Input: part model. Units: mm. Frame: model coordinates. Face numbers are marked on the shaded views. A direction names the side the tool comes from. Round coordinates to 2 decimals unless told otherwise and drop trailing zeros. Write each loop counter-clockwise with the first axis right and the second up, starting at its lowest first coordinate (ties: lowest second). Pieces come first, ordered by that corner, then holes. Notation, with made-up numbers: (41, 43) -> (48, 43) arc R31 cw to (48, 67) -> close; hole circle Ø7 at (53.5, -21.75). An arc over 180 degrees is marked (long way). Use CSV: the item, a comma, the result in double quotes.
```python
from build123d import *

# Parameters (mm, degrees)
SALIENTE_EXTRUIR1_DEPTH = 25.4
SALIENTE_EXTRUIR2_DEPTH = 12.7
CROQUIS4_R              = 3.96875
CORTAR_EXTRUIR2_DEPTH   = 143.085809608
REDONDEO1_SIZE          = 6.35


with BuildPart() as part:
    # Croquis1 → Saliente-Extruir1 (new, symmetric)
    with BuildSketch(Plane.XY):
        Polygon((21.5228, 45.6639), (31.367398371, 8.254586189), (0, 0), (-20, -40), (-123, -40), (-125, -38.012905156), (-125, -12.012905156), (-123.000083272, -10), (-65.000083272, -10), (-65.000083272, 15), (-107.993526537, 15), (-110, 16.993526537), (-110, 37.993526537), (-108.006473463, 40), (0, 40), align=None)
    extrude(amount=SALIENTE_EXTRUIR1_DEPTH, both=True)

    # Croquis2 → Saliente-Extruir2 (add, symmetric)
    with BuildSketch(Plane.XY):
        Polygon((29.677177015, 14.677399874), (92.537004524, 31.219530495), (86.072848866, 55.783216937), (23.213021357, 39.241086316), align=None)
    extrude(amount=SALIENTE_EXTRUIR2_DEPTH, both=True)

    # Croquis4 → Cortar-Extruir2 (cut, through all)
    with BuildSketch(Plane.XY.offset(12.7)):
        with Locations((72.381126981, 39.047723164)):
            Circle(CROQUIS4_R)
        with Locations((43.3688989, 31.412893647)):
            Circle(CROQUIS4_R)
    extrude(amount=-CORTAR_EXTRUIR2_DEPTH, mode=Mode.SUBTRACT)

    # Redondeo1
    redondeo1_edges = [part.edges().sort_by_distance(p)[0] for p in [
        (61.107090769, 22.948465184, -12.7),
        (54.642935111, 47.512151626, -12.7),
        (61.107090769, 22.948465184, 12.7),
        (54.642935111, 47.512151626, 12.7),
    ]]
    chamfer(redondeo1_edges, length=REDONDEO1_SIZE)


solid = part.part
```
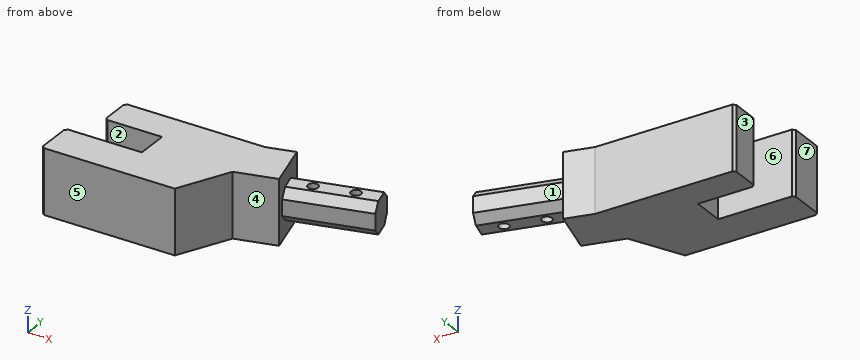
Item 1: Section query C-C on z = 16.5. Return the cut outline in (x, y), plus the area to 3 significant figures.
Worked answers:
outline,"(-125, -38.01) -> (-123, -40) -> (-20, -40) -> (0, 0) -> (31.37, 8.25) -> (21.52, 45.66) -> (0, 40) -> (-108.01, 40) -> (-110, 37.99) -> (-110, 16.99) -> (-107.99, 15) -> (-65, 15) -> (-65, -10) -> (-123, -10) -> (-125, -12.01) -> close"
area,"8,770 mm²"
Item 2: Section query D-D on x = 43. Return the cut outline in (y, z).
Worked answers:
outline,"(18.18, -6.35) -> (24.75, -12.7) -> (27.46, -12.7) -> (27.46, 12.7) -> (24.75, 12.7) -> (18.18, 6.35) -> close; (35.36, -12.7) -> (37.88, -12.7) -> (44.45, -6.35) -> (44.45, 6.35) -> (37.88, 12.7) -> (35.36, 12.7) -> close"
Item 3: Section query A-A on x = -80. Return the cut outline in (y, z).
Worked answers:
outline,"(-40, -25.4) -> (-10, -25.4) -> (-10, 25.4) -> (-40, 25.4) -> close; (15, -25.4) -> (40, -25.4) -> (40, 25.4) -> (15, 25.4) -> close"
Item 4: Line query: line 1 (Y direction, x = -99, z = -21.5); line 2 (Y direction, x = -24, z = 2); line 3 (Z direction, x = 74.5, y = 33). Output: solid intervals per line, ascending.
Worked answers:
line 1,"y = -40 to -10, 15 to 40"
line 2,"y = -40 to 40"
line 3,"z = -12.66 to 12.66"
Item 5: Pull-direction query (Y, two-part tool) for the marked faces 5, 6 and 7; classes: +Y half, -Y half, draft (parallel to the pull), parting line (faces both ways), or undercut.
Worked answers:
face 5,"-Y half"
face 6,"undercut"
face 7,"draft"
Item 6: Set-up query: the marked faces 1, 2, 3 and 4. Return all of +Z, -Z, +X, -X, +Y, -Y with unobstructed straight access to the full face (end or side cutting, diameter ignored); none if empty.
Worked answers:
face 1,"+Z, -Z, +Y"
face 2,"+Z, -Z, -X"
face 3,"+Z, -Z, -X, +Y"
face 4,"+Z, -Z, +X, -Y"
Item 7: Section query B-B on z = 4. Return the cut outline in (x, y).
Worked answers:
outline,"(-125, -38.01) -> (-123, -40) -> (-20, -40) -> (0, 0) -> (31.37, 8.25) -> (29.68, 14.68) -> (92.54, 31.22) -> (86.07, 55.78) -> (23.21, 39.24) -> (21.52, 45.66) -> (0, 40) -> (-108.01, 40) -> (-110, 37.99) -> (-110, 16.99) -> (-107.99, 15) -> (-65, 15) -> (-65, -10) -> (-123, -10) -> (-125, -12.01) -> close; hole circle Ø7.94 at (43.37, 31.41); hole circle Ø7.94 at (72.38, 39.05)"
Item 8: First-contact query: pin 1 Ø20 at (y, z) = (0.5, -11.5) entering from -X; pin 2 Ø1 at (x, z) = (-15, -15.5) entering from -Y; pin 3 Ø1 at (y, z) = (-21.5, -2.5) entering from +X; pin 4 Ø5 at (x, y) = (72.38, 39.05) entering from -Z. Flat tips, straight axial feed; report the tip coordinate or a pass-through.
Worked answers:
pin 1,"stops at x = -65"
pin 2,"stops at y = -31"
pin 3,"stops at x = -10.5"
pin 4,"passes through"
